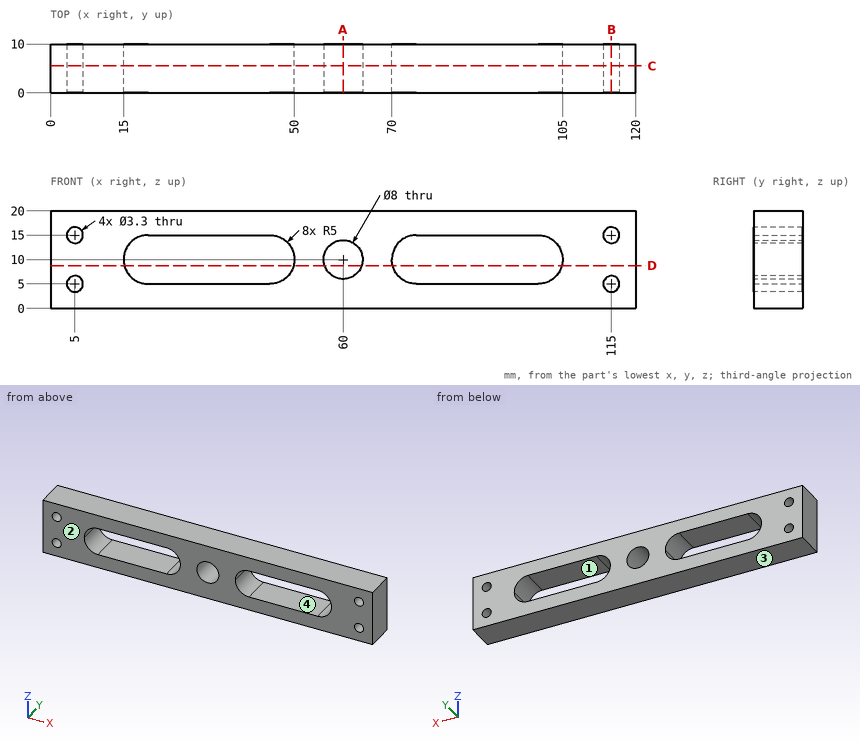
Geometry check sheet. Reference: drawing and pictorial views, mm from the part's lowest x, y, z. A direction names the side the tool comes from. Round coordinates to 2 decimals unless told otherwise and drop trailing zeros. Loops run counter-clockwise (first coordinate to the right, second up) from the corner with the lowest first, then second, coordinate; pieces in that order, holes last. Notation, with made-up numbers: (16.25, 56) - (42.25, 56) arc R21 ccw to (42.25, 92) - close; hole circle Ø8 at (47, 80). An arc over 180 degrees is marked (long way). Use a Markdown table: item, result. Add a question column.
1. Section check B-B, the plane x = 115. Record the boundary of the cut face in (y, z).
2. Access from +Z, -Z, +X, -X, +Y, -Y to the whole of each face (thin tool, end or side, straight path). Record for the marked faces 1 and 2.
3. Gauge pin test, flat end, axial feed: pin 1 (5 mm diameter, centred on x = 73.5, y = 7, fed in from -Z). Record the tip position at first contact, or that the pin passes through.
4. Section check D-D, the plane z = 8.75. Record the boundary of the cut face in (x, y).
5. Thickness scan on probe 1 along X at (y, z) = (6.5, 9.75); probe 2 along Z at (x, y) = (115, 7.5); probe 3 along Z at (x, y) = (88, 1.75). Record the ranges inside material, lowest first. Write a range as [from, to].
6. Section check C-C, the plane y = 5.5. Give the number of separate pieces and of enclosed holes in the cut face, plus the area to 3 significant figures.
7. Section check A-A, the plane x = 60. Record the boundary of the cut face in (y, z), plus the area to 3 significant figures.
8. Release check for a two-part mould opening along X. For the marked faces 3 and 4 record: released by +X, released by -X, zero draft, split by the parting line, or undercut.
Checks:
| question | item | result |
|---|---|---|
| 1 | outline | (0, 0) - (10, 0) - (10, 3.35) - (0, 3.35) - close; (0, 6.65) - (10, 6.65) - (10, 13.35) - (0, 13.35) - close; (0, 16.65) - (10, 16.65) - (10, 20) - (0, 20) - close |
| 2 | face 1 | +Y, -Y |
| 2 | face 2 | +Z, -Z, +X, -X, -Y |
| 3 | pin 1 | stops at z = 0 |
| 4 | outline | (0, 0) - (15.16, 0) - (15.16, 10) - (0, 10) - close; (49.84, 0) - (56.2, 0) - (56.2, 10) - (49.84, 10) - close; (63.8, 0) - (70.16, 0) - (70.16, 10) - (63.8, 10) - close; (104.84, 0) - (120, 0) - (120, 10) - (104.84, 10) - close |
| 5 | probe 1 | x = [0, 15.01], [49.99, 56.01], [63.99, 70.01], [104.99, 120] |
| 5 | probe 2 | z = [0, 3.35], [6.65, 13.35], [16.65, 20] |
| 5 | probe 3 | z = [0, 5], [15, 20] |
| 6 | separate pieces | 1 |
| 6 | enclosed holes | 7 |
| 6 | area | 1,660 mm^2 |
| 7 | outline | (0, 0) - (10, 0) - (10, 6) - (0, 6) - close; (0, 14) - (10, 14) - (10, 20) - (0, 20) - close |
| 7 | area | 120 mm^2 |
| 8 | face 3 | zero draft |
| 8 | face 4 | undercut |
